Build history of the part. All positions in model axes, mm. Face numbers are marked on the shaded views. A direction names the side the tool comes from. Round coordinates to 2 decimals unless told otherwise and drop trailing zeros. Loops run counter-clockwise (first coordinate to the right, second up) from the corner with the lowest first, then second, coordinate; pieces in that order, holes last. Notation, with made-up numbers: (-31, 35.5) - (-17, 35.5) arc R22 ccw to (-17, 51.5) - close; hole circle Ø11 at (-15.75, 86.5). An arc over 180 degrees is marked (long way). Put each result on its own line as item: value. Start each with the question number.
from build123d import *

# Parameters (mm, degrees)
SKETCH_1_W          = 20
SKETCH_1_H          = 5
EXTRUDE_1_DEPTH     = 35
SKETCH_2_W          = 30
SKETCH_2_H          = 20
EXTRUDE_2_DEPTH     = 3
FILLET_1_R          = 2
FILLET_2_R          = 2
FILLET_3_R          = 2
FILLET_4_R          = 2
SKETCH_4_W          = 30
SKETCH_4_H          = 40
EXTRUDE_3_DEPTH     = 2.5
FILLET_5_R          = 2
FILLET_6_R          = 2
CUT_EXTRUDE_2_DEPTH = 3
SKETCH_6_R          = 1.475
SKETCH_6_R_2        = 1.95
SKETCH_6_R_3        = 2.425
CUT_EXTRUDE_3_DEPTH = 3


with BuildPart() as part:
    # 草图1 → 凸台-拉伸1 (new body)
    with BuildSketch(Plane(origin=(0, 0, 0), x_dir=(0, 0, -1), z_dir=(1, 0, 0))):
        Rectangle(SKETCH_1_W, SKETCH_1_H)
    extrude(amount=-EXTRUDE_1_DEPTH)

    # 草图2 → 凸台-拉伸2 (add)
    with BuildSketch(Plane(origin=(0, 0, 0), x_dir=(0, 0, -1), z_dir=(1, 0, 0))):
        Rectangle(SKETCH_2_W, SKETCH_2_H)
    extrude(amount=EXTRUDE_2_DEPTH)

    # 圆角1
    fillet_1_edges = [part.edges().sort_by_distance(p)[0] for p in [
        (1.5, 10, -15),
    ]]
    fillet(fillet_1_edges, radius=FILLET_1_R)

    # 圆角2
    fillet_2_edges = [part.edges().sort_by_distance(p)[0] for p in [
        (1.5, 10, 15),
    ]]
    fillet(fillet_2_edges, radius=FILLET_2_R)

    # 圆角3
    fillet_3_edges = [part.edges().sort_by_distance(p)[0] for p in [
        (1.5, -10, -15),
    ]]
    fillet(fillet_3_edges, radius=FILLET_3_R)

    # 圆角4
    fillet_4_edges = [part.edges().sort_by_distance(p)[0] for p in [
        (1.5, -10, 15),
    ]]
    fillet(fillet_4_edges, radius=FILLET_4_R)

    # 草图4 → 凸台-拉伸3 (add, symmetric)
    with BuildSketch(Plane(origin=(0, 0, 0), x_dir=(1, 0, 0), z_dir=(0, 1, 0))):
        with Locations((-20, 0)):
            Rectangle(SKETCH_4_W, SKETCH_4_H)
    extrude(amount=EXTRUDE_3_DEPTH, both=True)

    # 圆角5
    fillet_5_edges = [part.edges().sort_by_distance(p)[0] for p in [
        (-5, 0, -10),
    ]]
    fillet(fillet_5_edges, radius=FILLET_5_R)

    # 圆角6
    fillet_6_edges = [part.edges().sort_by_distance(p)[0] for p in [
        (-5, 0, 10),
    ]]
    fillet(fillet_6_edges, radius=FILLET_6_R)

    # 草图5 → 切除-拉伸2 (cut)
    with BuildSketch(Plane(origin=(0, 0, 0), x_dir=(0, 0, -1), z_dir=(1, 0, 0))):
        with BuildLine():
            Line((-12, -1.5), (-15, -1.5))
            Line((-15, -1.5), (-15, 1.5))
            Line((-15, 1.5), (-12, 1.5))
            ThreePointArc((-12, 1.5), (-10.5, 0), (-12, -1.5))
        make_face()
        with BuildLine():
            Line((12, 1.5), (15, 1.5))
            Line((15, 1.5), (15, -1.5))
            Line((15, -1.5), (12, -1.5))
            ThreePointArc((12, -1.5), (10.5, 0), (12, 1.5))
        make_face()
    extrude(amount=CUT_EXTRUDE_2_DEPTH, mode=Mode.SUBTRACT)

    # 草图6 → 切除-拉伸3 (cut)
    with BuildSketch(Plane(origin=(0, 0, 0), x_dir=(0, 0, -1), z_dir=(1, 0, 0))):
        with Locations((0, -7)):
            Circle(SKETCH_6_R)
        with Locations((-7, -7)):
            Circle(SKETCH_6_R_2)
        with Locations((7, -7)):
            Circle(SKETCH_6_R_3)
        with Locations(Location((7, 7, 0), (0, 0, 180))):
            Circle(SKETCH_6_R_3)
        with Locations(Location((0, 7, 0), (0, 0, 180))):
            Circle(SKETCH_6_R)
        with Locations(Location((-7, 7, 0), (0, 0, 180))):
            Circle(SKETCH_6_R_2)
    extrude(amount=CUT_EXTRUDE_3_DEPTH, mode=Mode.SUBTRACT)


solid = part.part
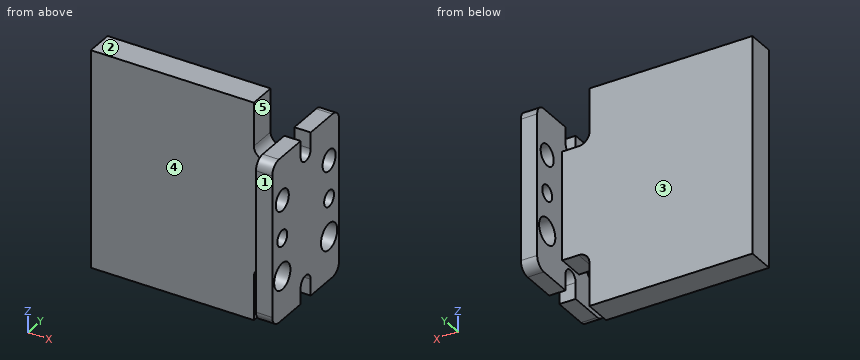
1) Drop flat-ended pins along their axis: pin 1 Ø10.5 at (x, z) = (-24.5, -3.5) entering from -Y; pin 2 Ø17.5 at (x, z) = (-26, -10) entering from +Y; pin 3 Ø0.9 at (x, y) = (1, -5) entering from -Z. Give the stop position or say it passes through.
2) Slice it at B-B, the plane y = 7. Write the cut outline in (x, z) (3 decimals).
3) Which spindle directions (+Z, -Z, +X, -X, +Y, -Y) get a long thin tool onto all of the face, cutting with end or side? Do the marked faces 1, 2, 3, 4 and 5. Say none if no direction does.
4) Slice it at A-A, the plane z = 0. Write the cut outline in (x, y) (3 decimals), and give its area (3 significant figures).
5) Slice it at D-D, the plane y = 3.75. Write the cut outline in (x, z).
6) Drill centre lines: line 1 (Y direction, x = 2.15, z = 7); line 2 (Y direction, x = 2.2, z = -7) (3 decimals); line 3 (Z direction, x = 2.45, y = 7) (3 decimals). Where is each one in solid material? Low to high. Write a range as [from, to].
7) Slice it at C-C, the plane x = -22. Write the cut outline in (y, z), and give its area (3 significant figures).
Taken from the geometry:
1. pin 1: stops at y = -2.5
1. pin 2: stops at y = 2.5
1. pin 3: stops at z = -15
2. outline: (0, -15) - (3, -15) - (3, -9.425) - (0, -9.425) - close; (0, -4.575) - (3, -4.575) - (3, -1.475) - (0, -1.475) - close; (0, 1.475) - (3, 1.475) - (3, 5.05) - (0, 5.05) - close; (0, 8.95) - (3, 8.95) - (3, 15) - (0, 15) - close
3. face 1: +Z, -Z, +X, -X, -Y
3. face 2: +Z, +X, -X, +Y, -Y
3. face 3: +Z, -Z, -X, +Y
3. face 4: +Z, -Z, -X, -Y
3. face 5: +Z, +Y, -Y
4. outline: (-35, -2.5) - (0, -2.5) - (0, -5.525) - (3, -5.525) - (3, 5.525) - (0, 5.525) - (0, 2.5) - (-35, 2.5) - close; (0, -10) - (3, -10) - (3, -8.475) - (0, -8.475) - close; (0, 8.475) - (3, 8.475) - (3, 10) - (0, 10) - close
4. area: 217 mm2
5. outline: (0, -15) - (3, -15) - (3, 15) - (0, 15) - close
6. line 1: y = [-10, -8.95], [-5.05, 5.05], [8.95, 10]
6. line 2: y = [-10, -9.425], [-4.575, 4.575], [9.425, 10]
6. line 3: z = [-15, -9.425], [-4.575, -1.475], [1.475, 5.05], [8.95, 15]
7. outline: (-2.5, -20) - (2.5, -20) - (2.5, 20) - (-2.5, 20) - close
7. area: 200 mm2
